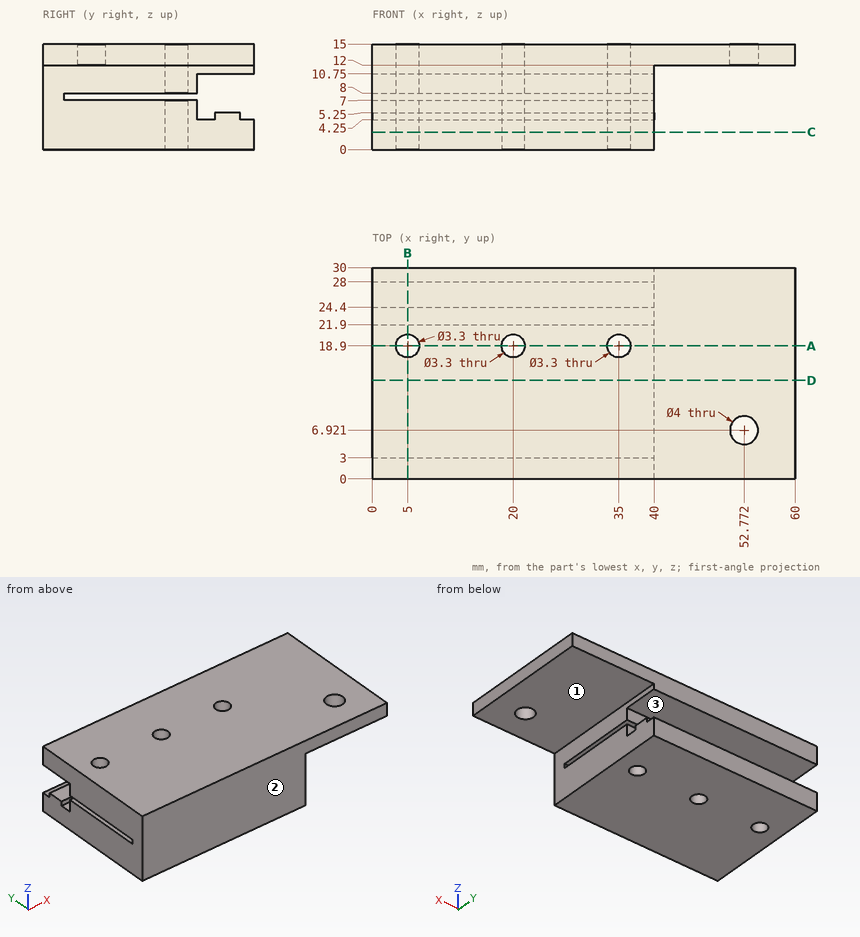
Here's the drawing with two shaded views (mm, measured from the low corner). I have some questions. A direction names the side the tool comes from. Coordinates: 2 decimals unless noted, no trailing zeros. Write each loop counter-clockwise with the first axis right and the second up, starting at its lowest first coordinate (ties: lowest second). Pieces come first, ordered by that corner, then holes.
Item 1: If I drill on line 1 (X direction, y = 18.9, z = 2); line 2 (Y direction, x = 35, z = 4.5); line 3 (Z direction, x = 27, y = 21.75), over which ranges is the centre line in solid material (lowest first)?
Item 2: I want a section at C-C on z = 2.5. Write out the boundary of the cut face in (x, y), and give its area (3 significant figures).
Item 3: On a 3-axis mill with a long thin cutter (end or side, diameter ignored), from which of +Z, -Z, +X, -X, +Y, -Y can I reach the whole of each face in a straight line? I mean the marked faces 1, 2 and 3. Say none if no direction works.
Item 4: Will these pins go through, and if not, where does the flat tip stop? pin 1 (1.5 mm diameter, centred on x = 52.5, y = 10.5, fed in from -Z); pin 2 (2 mm diameter, centred on y = 25, z = 2.5, fed in from +X); pin 3 (0.8 mm diameter, centred on x = 10.5, z = 7.5, fed in from +Y).
Item 5: I want a section at D-D on y = 14. Write out the boundary of the cut face in (x, z).
Item 6: I want a section at B-B on x = 5. Write out the boundary of the cut face in (y, z), and give its area (3 significant figures).
Item 7: I want a section at A-A on y = 18.9. Count the separate pieces of the cut face and the enclosed holes in it.
Findings below:
1. line 1: x = 0 to 3.35, 6.65 to 18.35, 21.65 to 33.35, 36.65 to 40
1. line 2: y = 0 to 17.25, 20.55 to 21.9, 24.4 to 28
1. line 3: z = 0 to 7, 8 to 15
2. outline: (0, 0) - (40, 0) - (40, 30) - (0, 30) - close; hole circle Ø3.3 at (5, 18.9); hole circle Ø3.3 at (20, 18.9); hole circle Ø3.3 at (35, 18.9)
2. area: 1,170 mm2
3. face 1: -Z, +X, +Y, -Y
3. face 2: +Z, -Z, +X, -X, -Y
3. face 3: +X, -X, +Y
4. pin 1: stops at z = 12
4. pin 2: stops at x = 40
4. pin 3: stops at y = 3
5. outline: (0, 0) - (40, 0) - (40, 7) - (0, 7) - close; (0, 8) - (40, 8) - (40, 12) - (60, 12) - (60, 15) - (0, 15) - close
6. outline: (0, 0) - (17.25, 0) - (17.25, 7) - (3, 7) - (3, 8) - (17.25, 8) - (17.25, 15) - (0, 15) - close; (20.55, 0) - (30, 0) - (30, 4.25) - (28, 4.25) - (28, 5.25) - (24.4, 5.25) - (24.4, 4.25) - (21.9, 4.25) - (21.9, 7) - (20.55, 7) - close; (20.55, 8) - (21.9, 8) - (21.9, 10.75) - (30, 10.75) - (30, 15) - (20.55, 15) - close
6. area: 336 mm2
7. separate pieces: 8
7. enclosed holes: 0
